Input: part model. Units: mm. Frame: model coordinates. A direction names the side the tool comes from. Round coordinates to 2 decimals unless told otherwise and drop trailing zeros. Order: outer loops, then holes, each group sorted by start corner. A loop starts at its lowest first (then second) coordinate and runs counter-clockwise, first axis right, second up. Notation, with made-up numbers: (7, 45.25) -> (15, 45.25) arc R37 ccw to (15, 81.25) -> close; hole circle Ø11 at (29.5, 84.5). An arc over 180 degrees is marked (long way). Use a Markdown table: item, result.
from build123d import *

# Parameters (mm, degrees)
F0_R     = 39.000467
F1_DEPTH = 55.626
F2_R     = 21.469452
F3_DEPTH = 29.464
F4_R     = 19.490474
F5_DEPTH = 25.4
F6_R     = 56.331947
F7_DEPTH = 68.834
F8_R     = 6.495267
F9_DEPTH = 169.164


with BuildPart() as f1:
    # F0 (on Top) → F1 (new body)
    with BuildSketch(Plane.XY):
        Circle(F0_R)
    extrude(amount=F1_DEPTH)

    # F2 (on face) → F3 (join)
    with BuildSketch(Plane.XY.offset(55.626)):
        Circle(F2_R)
    extrude(amount=-F3_DEPTH)

    # F4 (on face) → F5 (cut)
    with BuildSketch(Plane.XY.offset(55.626)):
        Circle(F4_R)
    extrude(amount=-F5_DEPTH, mode=Mode.SUBTRACT)

    # F6 (on face) → F7 (join)
    with BuildSketch(Plane(origin=(0, 0, 0), x_dir=(1, 0, 0), z_dir=(0, 0, -1))):
        Circle(F6_R)
    extrude(amount=F7_DEPTH)

    # F8 (on face) → F9 (cut)
    with BuildSketch(Plane.XY.offset(30.226)):
        Circle(F8_R)
    extrude(amount=-F9_DEPTH, mode=Mode.SUBTRACT)


solid = f1.part
1) Pull-direction query (X, two-part tool) for faces 1 (the cylindrical face through (-7.333, -55.853, -33.935)), 2 (the flat face through (12, -1, -68.834)), 3 (the cylindrical face through (6.195, 1.951, -18.611)); classes: +X half, -X half, draft (parallel to the pull), parting line (faces both ways), or undercut.
Results found:
| item | result |
|---|---|
| face 1 | parting line |
| face 2 | draft |
| face 3 | undercut |
2) Line query: L1, parallel to Y at x = 0, z = 45; L2, parallel to Y at x = 0, z = -9; L3, parallel to Z at x = -33, y = 37.5. Output: solid intervals per line, ascending. Write a range as [from, to].
Results found:
| item | result |
|---|---|
| L1 | y = [-39, -19.49], [19.49, 39] |
| L2 | y = [-56.33, -6.5], [6.5, 56.33] |
| L3 | z = [-68.83, 0] |
3) Cut plane C-C on z = -34. Return loops of the section in (x, y).
Results found:
| item | result |
|---|---|
| outline | circle Ø112.66 at (0, 0); hole circle Ø12.99 at (0, 0) |
4) Pin query (flat end, axial travel): pin 1 Ø1.5 at (y, z) = (30.5, 20.5) entering from +X; pin 2 Ø2 at (x, z) = (36.5, -46) entering from -Y; pin 3 Ø4 at (x, z) = (-36.5, -12.5) entering from -Y; pin 4 Ø8 at (x, y) = (0, 0) entering from +Z. Return the tip coordinate at first contact, or that it passes through.
Results found:
| item | result |
|---|---|
| pin 1 | stops at x = 25.22 |
| pin 2 | stops at y = -43.74 |
| pin 3 | stops at y = -44.53 |
| pin 4 | passes through |
5) Cut plane D-D on x = 28.5. Return loops of the section in (y, z).
Results found:
| item | result |
|---|---|
| outline | (-48.59, -68.83) -> (48.59, -68.83) -> (48.59, 0) -> (26.62, 0) -> (26.62, 55.63) -> (-26.62, 55.63) -> (-26.62, 0) -> (-48.59, 0) -> close |
6) Set-up query: faces 4 (the flat face through (-18, -8, 55.626)), 5 (the flat face through (-5, 5, 30.226)). Return all of +Z, -Z, +X, -X, +Y, -Y with unobstructed straight access to the full face (end or side cutting, diameter ignored); none if empty.
Results found:
| item | result |
|---|---|
| face 4 | +Z, +X, -X, +Y, -Y |
| face 5 | +Z |
7) Cut plane A-A on y = 0. Return loops of the section in (x, z).
Results found:
| item | result |
|---|---|
| outline | (-56.33, -68.83) -> (-6.5, -68.83) -> (-6.5, 30.23) -> (-19.49, 30.23) -> (-19.49, 55.63) -> (-39, 55.63) -> (-39, 0) -> (-56.33, 0) -> close; (6.5, -68.83) -> (56.33, -68.83) -> (56.33, 0) -> (39, 0) -> (39, 55.63) -> (19.49, 55.63) -> (19.49, 30.23) -> (6.5, 30.23) -> close |
